from build123d import *


with BuildPart() as f1:
    # F0 (on Front) → F1 (revolve)
    with BuildSketch(Plane.XZ):
        with BuildLine():
            Line((211.396159, 8.87954), (7.905546, 15.811093))
            Line((7.905546, 15.811093), (0, 15.811093))
            Line((0, 15.811093), (0, -17.851226))
            Line((0, -17.851226), (7.905546, -17.851226))
            Line((7.905546, -17.851226), (211.457818, -8.936529))
            ThreePointArc((211.457818, -8.936529), (215.767289, -6.983409), (217.529982, -2.59261))
            Line((217.529982, -2.59261), (217.529982, 2.533221))
            ThreePointArc((217.529982, 2.533221), (215.745901, 6.946257), (211.396159, 8.87954))
        make_face()
    revolve(axis=Axis((0, 0, -1.020066), (0, 0, 1)))


solid = f1.part
CAD build for the part. Positions are in the model's coordinates, mm. Give positions to 0.01 mm unless a question says otherwise; leave off trailing zeros. Loops run counter-clockwise (first coordinate to the right, second up) from the corner with the lowest first, then second, coordinate; pieces in that order, holes last. Notation, with made-up numbers: M 3,-20.5 L 48,-20.5 A26 cw 48,1.5 Z; hole C -6,72.25 d11. An arc over 180 degrees is marked long. One line per question, with ' | ' between items. Start each with the question number.
1. Two-plate mould, pull along Z, no slides. Class faces 1 (the face through (-47.156, -212.357, 0.006)), 2 (the face through (0, 0, -17.851)), 3 (the face through (16.965, 5.342, 15.475)): pulls with the +Z half, pulls with the -Z half, needs draft (parallel to the pull), parting line crosses it, or undercut.
2. Probe L1, parallel to Y at x = 171.5, z = 4.5; L2, parallel to X at y = 93, z = -4; L3, parallel to Y at x = 112.5, z = 3.5. List the from-to ranges inside material, lowest first. Write a range as from..to.
3. Flat gauge pins, fed straight in: pin 1 (10 mm diameter, centred on x = 154.5, z = 2.5, fed in from +Y); pin 2 (8 mm diameter, centred on x = -64, z = -2.5, fed in from +Y); pin 3 (6 mm diameter, centred on x = 171.5, y = 61.5, fed in from +Z). Where does each tip first touch, or does it go through?
4. Saw through at A-A on x = 0. Give the cut face in (y, z).
Result sheet:
1) face 1: needs draft | face 2: pulls with the -Z half | face 3: pulls with the +Z half
2) L1: y = -133.31..133.31 | L2: x = -196.47..196.47 | L3: y = -186.09..186.09
3) pin 1: stops at y = 158.02 | pin 2: stops at y = 209.09 | pin 3: stops at z = 9.98
4) outline: M -217.53,-2.59 A6.35 ccw -211.46,-8.94 L -7.91,-17.85 L 7.91,-17.85 L 211.46,-8.94 A6.35 ccw 217.53,-2.59 L 217.53,2.53 A6.35 ccw 211.4,8.88 L 7.91,15.81 L -7.91,15.81 L -211.4,8.88 A6.35 ccw -217.53,2.53 Z
